Input: part model. Units: mm. Frame: model coordinates. Give positions to 0.01 mm unless a question says otherwise; leave off trailing zeros. Loops run counter-clockwise (first coordinate to the right, second up) from the corner with the lowest first, then second, coordinate; pieces in that order, holes last. Notation, with made-up numbers: (-1, 1) - (40, 1) arc R32 ccw to (40, 35) - close; hole circle Ø2 at (63.25, 36). An arc over 180 degrees is marked (long way). Answer as a JSON object with one key per item and string values. Group by question number.
(1) Section query A-A (y = 10.5). Return loops of the section in (x, z) (3 decimals).
(2) Section query B-B (x = -78). Return loops of the section in (y, z).
(3) Pin query (flat end, axial travel): P1, Ø1, axis at x = -11.5, y = -2.5, coming from the -Z side; P2, Ø9.5, axis at x = -32, y = 11.5, coming from the -Z side; P3, Ø9.5, axis at x = -16.5, y = 7.5, coming from the +Z side. Return the tip coordinate at first contact, or that it passes through.
(4) Material intervals for L1, parallel to Z at x = -46, y = 10.5; L2, parallel to Z at x = 30.5, y = 12; L3, parallel to Y at x = -30, z = 817, sorted ascending.
```python
from build123d import *

# Parameters (mm, degrees)
F0_W     = 184.15
F0_H     = 38.1
F1_DEPTH = 1625.6
F3_DEPTH = 190.5
F4_W     = 184.15
F4_H     = 38.1
F5_DEPTH = 19.05


with BuildPart() as f1:
    # F0 (on Top) → F1 (new body)
    with BuildSketch(Plane.XY):
        Rectangle(F0_W, F0_H)
    extrude(amount=F1_DEPTH)

    # F2 (on face) → F3 (cut)
    with BuildSketch(Plane.YZ.offset(92.075)):
        Polygon((19.05, 1625.6), (-19.05, 1625.6), (19.05, 1587.5), align=None)
        Polygon((19.05, 38.1), (-19.05, 0), (19.05, 0), align=None)
    extrude(amount=-F3_DEPTH, mode=Mode.SUBTRACT)

    # F4 (on face) → F5 (cut)
    with BuildSketch(Plane(origin=(0, 19.05, 0), x_dir=(-1, 0, 0), z_dir=(0, 1, 0))):
        with Locations((0, 812.8)):
            Rectangle(F4_W, F4_H)
    extrude(amount=-F5_DEPTH, mode=Mode.SUBTRACT)


solid = f1.part
```
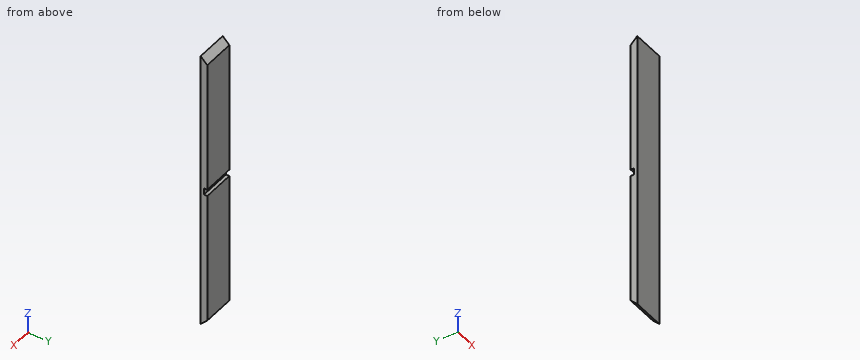
Recorded:
{
 "1": {"outline": "(-92.075, 29.55) - (92.075, 29.55) - (92.075, 793.75) - (-92.075, 793.75) - close; (-92.075, 831.85) - (92.075, 831.85) - (92.075, 1596.05) - (-92.075, 1596.05) - close"},
 "2": {"outline": "(-19.05, 0) - (19.05, 38.1) - (19.05, 793.75) - (0, 793.75) - (0, 831.85) - (19.05, 831.85) - (19.05, 1587.5) - (-19.05, 1625.6) - close"},
 "3": {"P1": "stops at z = 16.05", "P2": "stops at z = 25.8", "P3": "stops at z = 1603.8"},
 "4": {"L1": "z = 29.55 to 793.75, 831.85 to 1596.05", "L2": "z = 31.05 to 793.75, 831.85 to 1594.55", "L3": "y = -19.05 to 0"}
}
